from build123d import *

# Parameters (mm, degrees)
SKETCH1_W           = 24.9682
SKETCH1_H           = 17.1704
BOSS_EXTRUDE1_DEPTH = 4.2926
SKETCH3_W           = 12.0015
SKETCH3_H           = 4.4577
BOSS_EXTRUDE2_DEPTH = 9.7536
SKETCH4_R           = 1.27
BOSS_EXTRUDE3_DEPTH = 2.54


with BuildPart() as part:
    # Sketch1 → Boss-Extrude1 (new, symmetric)
    with BuildSketch(Plane(origin=(0, 0, 0), x_dir=(1, 0, 0), z_dir=(0, 1, 0))):
        Rectangle(SKETCH1_W, SKETCH1_H)
    extrude(amount=BOSS_EXTRUDE1_DEPTH, both=True)

    # Sketch3 → Boss-Extrude2 (add)
    with BuildSketch(Plane(origin=(12.4841, 0, 0), x_dir=(0, 0, -1), z_dir=(1, 0, 0))):
        Rectangle(SKETCH3_W, SKETCH3_H)
    extrude(amount=BOSS_EXTRUDE2_DEPTH)

    # Sketch4 → Boss-Extrude3 (add)
    with BuildSketch(Plane.ZY.offset(12.4841)):
        with Locations(Location((0, 0, 0), (0, 0, 180))):
            Circle(SKETCH4_R)
    extrude(amount=BOSS_EXTRUDE3_DEPTH)


solid = part.part
CAD build for the part. Positions are in the model's coordinates, mm. A direction names the side the tool comes from. Round coordinates to 2 decimals unless told otherwise and drop trailing zeros. Write each loop counter-clockwise with the first axis right and the second up, starting at its lowest first coordinate (ties: lowest second). Pieces come first, ordered by that corner, then holes.
(1) Probe line 1 along X through (y, z) = (-1, -5.25); line 2 along X through (y, z) = (2.5, 3.75); line 3 along Y through (x, z) = (14, -3.75). List the from-to ranges inside material, lowest first.
(2) Slice it at B-B, the plane z = 0. Write the cut outline in (x, y).
(3) Drop flat-ended pins along their axis: P1, Ø5, axis at x = 17.5, y = 1, coming from the -Z side; P2, Ø1.3, axis at x = 16, y = 0, coming from the +Z side; P3, Ø3, axis at x = 15.5, z = 4, coming from the -Y side; P4, Ø4.5, axis at y = 2, z = 1, coming from the -X side. Give the stop position or say it passes through.
(4) 3-axis set-ups, long thin cutter, end or side, ignore diameter. For faces 1 (the face through (17, -2.229, 0)), 2 (the face through (17, 2.229, 0)), 3 (the face through (-13.74, -1.26, 0.17)): which of +Z, -Z, +X, -X, +Y, -Y reach the whole face in a straight line?
(5) Slice it at A-A, the plane y = -1.75. Write the cut outline in (x, z), and give its area (3 significant figures).
(6) Slice it at D-D, the plane z = -1.75. Write the cut outline in (x, y), and give its area (3 significant figures).
(7) Slice it at C-C, the plane y = 0. Write the cut outline in (x, z).
From the geometry:
1. line 1: x = -12.48 to 22.24
1. line 2: x = -12.48 to 12.48
1. line 3: y = -2.23 to 2.23
2. outline: (-15.02, -1.27) - (-12.48, -1.27) - (-12.48, -4.29) - (12.48, -4.29) - (12.48, -2.23) - (22.24, -2.23) - (22.24, 2.23) - (12.48, 2.23) - (12.48, 4.29) - (-12.48, 4.29) - (-12.48, 1.27) - (-15.02, 1.27) - close
3. P1: stops at z = -6
3. P2: stops at z = 6
3. P3: stops at y = -2.23
3. P4: stops at x = -15.02
4. face 1: +Z, -Z, +X, -Y
4. face 2: +Z, -Z, +X, +Y
4. face 3: -X
5. outline: (-12.48, -8.59) - (12.48, -8.59) - (12.48, -6) - (22.24, -6) - (22.24, 6) - (12.48, 6) - (12.48, 8.59) - (-12.48, 8.59) - close
5. area: 546 mm2
6. outline: (-12.48, -4.29) - (12.48, -4.29) - (12.48, -2.23) - (22.24, -2.23) - (22.24, 2.23) - (12.48, 2.23) - (12.48, 4.29) - (-12.48, 4.29) - close
6. area: 258 mm2
7. outline: (-15.02, -1.27) - (-12.48, -1.27) - (-12.48, -8.59) - (12.48, -8.59) - (12.48, -6) - (22.24, -6) - (22.24, 6) - (12.48, 6) - (12.48, 8.59) - (-12.48, 8.59) - (-12.48, 1.27) - (-15.02, 1.27) - close
